Could you check a few things on this drawing? It's one solid part, dimensions in mm from its lowest x, y, z. A direction names the side the tool comes from. Give positions to 0.01 mm unless a question says otherwise; leave off trailing zeros. Loops run counter-clockwise (first coordinate to the right, second up) from the corner with the lowest first, then second, coordinate; pieces in that order, holes last. Notation, with made-up numbers: (-7.75, 82.25) -> (41.25, 82.25) arc R13 ccw to (41.25, 96.25) -> close; hole circle Ø9 at (21.5, 56.25). An arc over 180 degrees is marked (long way). One line per question, with ' | ' between items.
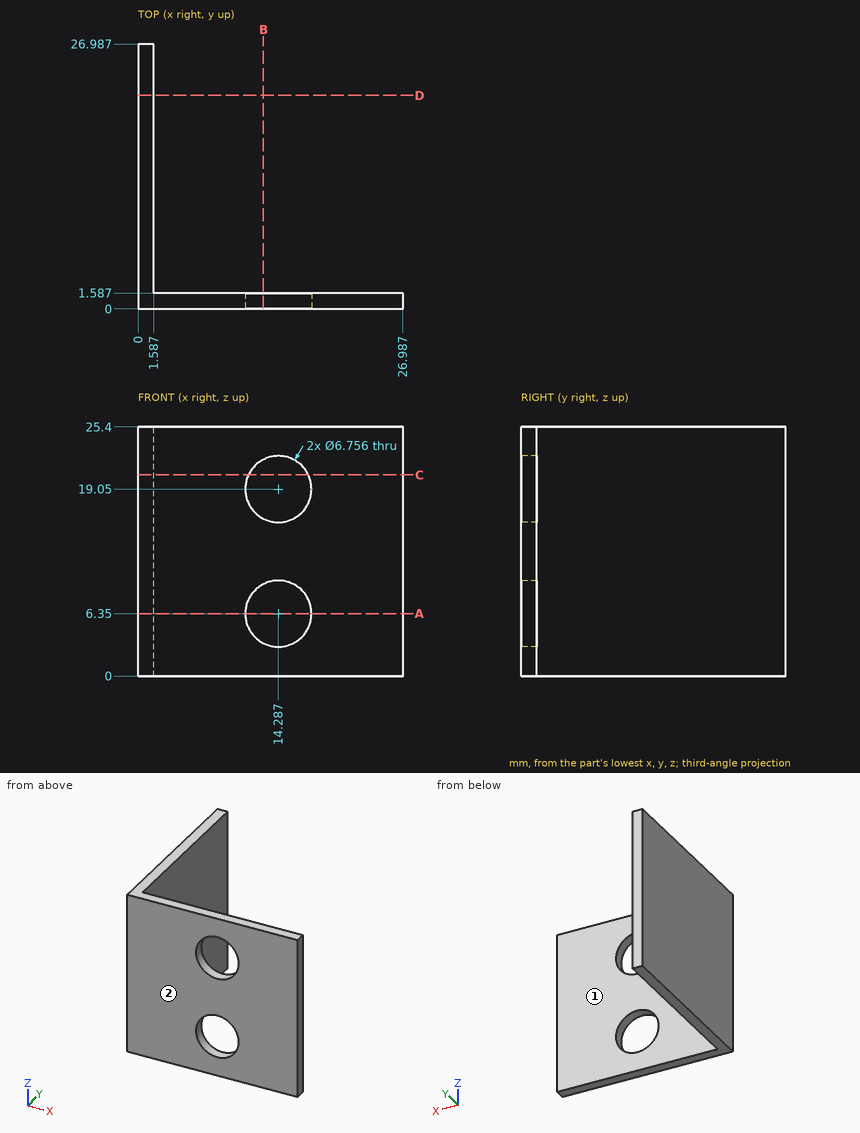
Q1. For pin 1 Ø11 at (x, z) = (14.29, 19.05) entering from +Y; pin 2 Ø1 at (y, z) = (19, 11.5) entering from +X; pin 3 Ø5.5 at (x, z) = (14.29, 6.35) entering from -Y, each with a flat end and sliding along its axis, tell me the tip position at first contact or that it passes through.
Entries:
pin 1: y = 1.59 | pin 2: x = 1.59 | pin 3: through
Q2. If we section it at B-B (x = 12.75): Write out the boundary of the cut face in (y, z).
Entries:
outline: (0, 0) -> (1.59, 0) -> (1.59, 3.34) -> (0, 3.34) -> close; (0, 9.36) -> (1.59, 9.36) -> (1.59, 16.04) -> (0, 16.04) -> close; (0, 22.06) -> (1.59, 22.06) -> (1.59, 25.4) -> (0, 25.4) -> close
Q3. On a 3-axis mill with a long thin cutter (end or side, diameter ignored), from which of +Z, -Z, +X, -X, +Y, -Y can I reach the whole of each face in a straight line? I mean the marked faces 1 and 2. Say none if no direction works.
Entries:
face 1: +Z, -Z, +X, +Y | face 2: +Z, -Z, +X, -X, -Y
Q4. If we section it at A-A (z = 6.35): Write out the boundary of the cut face in (x, y) (1 decimal).
Entries:
outline: (0, 0) -> (10.9, 0) -> (10.9, 1.6) -> (1.6, 1.6) -> (1.6, 27) -> (0, 27) -> close; (17.7, 0) -> (27, 0) -> (27, 1.6) -> (17.7, 1.6) -> close
Q5. If we section it at D-D (y = 21.75): Write out the boundary of the cut face in (x, z).
Entries:
outline: (0, 0) -> (1.59, 0) -> (1.59, 25.4) -> (0, 25.4) -> close
Q6. If we section it at C-C (z = 20.5): Write out the boundary of the cut face in (x, y).
Entries:
outline: (0, 0) -> (11.24, 0) -> (11.24, 1.59) -> (1.59, 1.59) -> (1.59, 26.99) -> (0, 26.99) -> close; (17.34, 0) -> (26.99, 0) -> (26.99, 1.59) -> (17.34, 1.59) -> close
Q7. If I drill on probe 1 along X at (y, z) = (0.6, 19.05) (1 decimal); probe 2 along Y at (x, z) = (18.25, 21.5), over which ranges is the centre line in solid material (lowest first)? Write a range as from..to.
Entries:
probe 1: 0..10.9, 17.7..27 | probe 2: 0..1.59
